from build123d import *

# Parameters (mm, degrees)
SKETCH1_R           = 2.75
BOSS_EXTRUDE1_DEPTH = 5


with BuildPart() as part:
    # Sketch1 → Boss-Extrude1 (new body)
    with BuildSketch(Plane.XY):
        with BuildLine():
            Line((0, 5), (0, 10))
            ThreePointArc((0, 10), (1.464466094, 13.535533906), (5, 15))
            Line((5, 15), (75, 15))
            ThreePointArc((75, 15), (78.535533906, 13.535533906), (80, 10))
            Line((80, 10), (80, 5))
            ThreePointArc((80, 5), (78.535533906, 1.464466094), (75, 0))
            Line((75, 0), (5, 0))
            ThreePointArc((5, 0), (1.464466094, 1.464466094), (0, 5))
        make_face()
        with Locations((7.5, 7.5)):
            Circle(SKETCH1_R, mode=Mode.SUBTRACT)
        with BuildLine():
            Line((42.5, 12.55), (72, 12.55))
            ThreePointArc((72, 12.55), (77.05, 7.5), (72, 2.45))
            Line((72, 2.45), (42.5, 2.45))
            ThreePointArc((42.5, 2.45), (37.45, 7.5), (42.5, 12.55))
        make_face(mode=Mode.SUBTRACT)
    extrude(amount=BOSS_EXTRUDE1_DEPTH)


solid = part.part
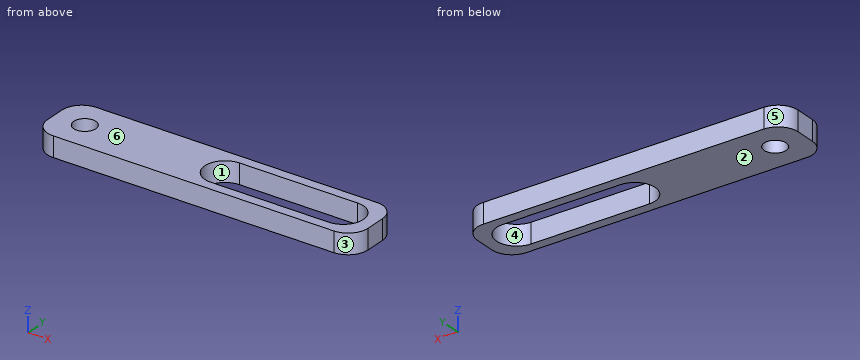
Design review of the part built by this model. Coordinates are the model's own, in mm. Face numbers are marked on the shaded views. A direction names the side the tool comes from. Give positions to 0.01 mm unless a question says otherwise; leave off trailing zeros. Loops run counter-clockwise (first coordinate to the right, second up) from the corner with the lowest first, then second, coordinate; pieces in that order, holes last. Notation, with made-up numbers: M 72.5,-33 L 101.5,-33 A22 ccw 101.5,-21 Z; hole C 85.25,6 d10. An arc over 180 degrees is marked long. Answer as a JSON object with one key per item and string values.
Item 1: We need section B-B (z = 0.95). State the section outline as (x, y) points.
Output values:
{"outline": "M 0,5 A5 ccw 5,0 L 75,0 A5 ccw 80,5 L 80,10 A5 ccw 75,15 L 5,15 A5 ccw 0,10 Z; hole C 7.5,7.5 d5.5; hole M 42.5,2.45 L 72,2.45 A5.05 ccw 72,12.55 L 42.5,12.55 A5.05 ccw Z"}
Item 2: Wall thickness on line 1 along X through (y, z) = (7.25, 2.1); line 2 along Y through (x, z) = (7.5, 1.45); line 3 along X through (y, z) = (9.75, 4.8): over which ranges is each line inside the solid? List them lowest first.
Output values:
{"line 1": "x = 0 to 4.76, 10.24 to 37.46, 77.04 to 80", "line 2": "y = 0 to 4.75, 10.25 to 15", "line 3": "x = 0 to 5.92, 9.08 to 37.98, 76.52 to 80"}
Item 3: Machinability: for the marked faces 1 and 2, which of the approach directions +Z, -Z, +X, -X, +Y, -Y give a long, thin tool a straight path to every point of the face, cutting with its end or side? Answer none if there is none.
Output values:
{"face 1": "+Z, -Z", "face 2": "-Z, +X, -X, +Y, -Y"}
Item 4: For P1, Ø3, axis at x = 49.5, y = 5.5, coming from the +Z side, flat-tipped, find the tip position at first contact; note if it passes through.
Output values:
{"P1": "passes through"}
Item 5: Mouldability with a two-part tool opening along X and no side actions: class the marked faces 3, 4, 5 and 6 as pulls with the +X half, pulls with the -X half, needs draft (parallel to the pull), parting line crosses it, or undercut.
Output values:
{"face 3": "pulls with the +X half", "face 4": "undercut", "face 5": "pulls with the -X half", "face 6": "needs draft"}
Item 6: We need section D-D (x = 68.5). State the section outline as (y, z) points, and give its area (3 significant figures).
Output values:
{"outline": "M 0,0 L 2.45,0 L 2.45,5 L 0,5 Z; M 12.55,0 L 15,0 L 15,5 L 12.55,5 Z", "area": "24.5 mm2"}
Item 7: We need section C-C (y = 7.5). State the section outline as (x, z) points.
Output values:
{"outline": "M 0,0 L 4.75,0 L 4.75,5 L 0,5 Z; M 10.25,0 L 37.45,0 L 37.45,5 L 10.25,5 Z; M 77.05,0 L 80,0 L 80,5 L 77.05,5 Z"}
Item 8: We need section A-A (x = 7.5). State the section outline as (y, z) points.
Output values:
{"outline": "M 0,0 L 4.75,0 L 4.75,5 L 0,5 Z; M 10.25,0 L 15,0 L 15,5 L 10.25,5 Z"}
